Study the drawing (mm; zero at the part's minimum x, y, z) and answer. Round coordinates to 2 decimals unless told otherwise and drop trailing zeros. Loops run counter-clockwise (first coordinate to the right, second up) from the corner with the lowest first, then second, coordinate; pieces in that order, holes last. Notation, with made-up numbers: M -34.75,42 L -11.75,42 A6 ccw -11.75,49 Z; hole C 6.5,73 d5. An arc over 180 degrees is marked long. Put each result on its own line as item: value. Start each with the question number.
(1) Straight lines are drawn through the part: line 1 (X direction, y = 3.55, z = 130); line 2 (X direction, y = 3.2, z = 143.5); line 3 (Z direction, x = 28.5, y = 0.4). For each, find the intervals that lie inside material, in ascending order.
(2) Section C-C, the plane x = 22.5 is taken. Determine the outline of the cut face in (y, z).
(3) Section D-D, the plane x = 28.25 is taken. Determine the outline of the cut face in (y, z).
(4) Section A-A, the plane z = 130 is taken. Determine the outline of the cut face in (x, y), then the cut area to 3 significant figures.
(5) A flat-ended cylindrical pin translates along its axis: P1, Ø4.5, axis at x = 22.5, z = 115, coming from the +Y side. Find the tip coordinate at first contact, or state that the pin passes through.
(6) Section B-B, the plane y = 2.8 is taken. Count the separate pieces of the cut face and the enclosed holes in it, then the cut area to 3 significant figures.
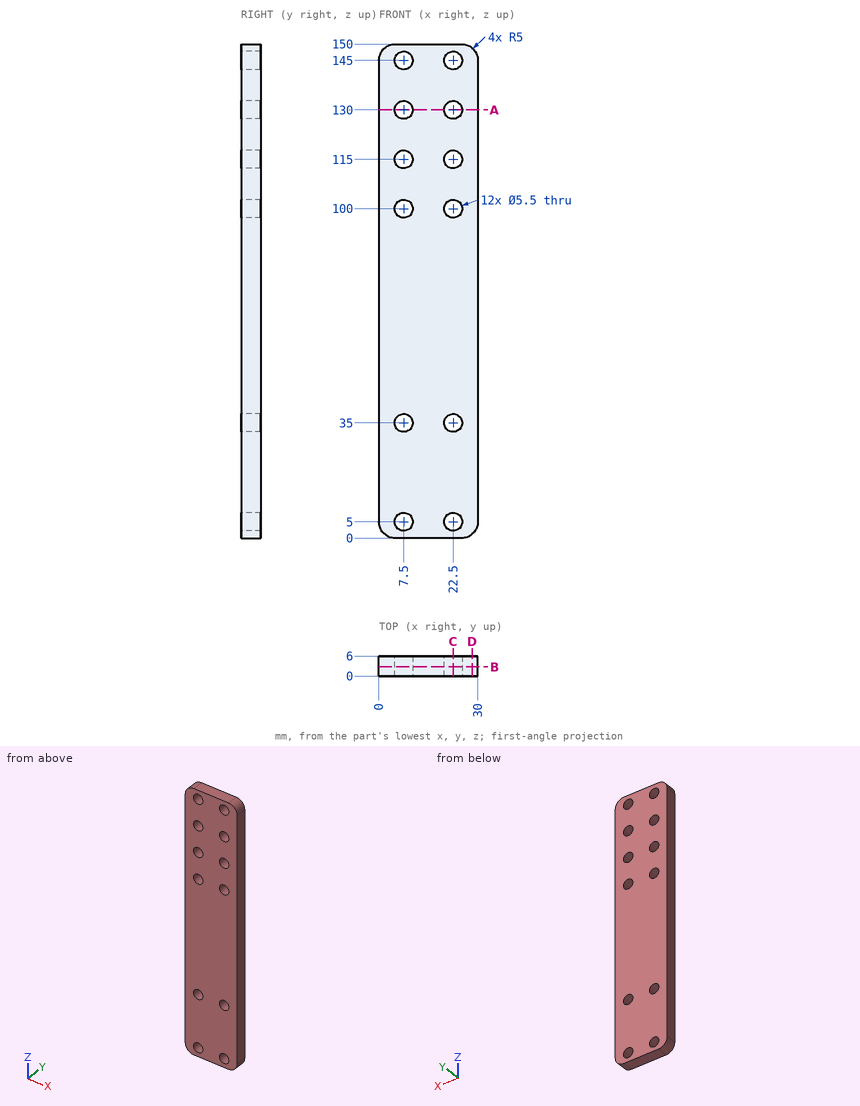
Recorded:
1. line 1: x = 0 to 4.75, 10.25 to 19.75, 25.25 to 30
1. line 2: x = 0 to 5.2, 9.8 to 20.2, 24.8 to 30
1. line 3: z = 1.43 to 148.57
2. outline: M 0,0 L 6,0 L 6,2.25 L 0,2.25 Z; M 0,7.75 L 6,7.75 L 6,32.25 L 0,32.25 Z; M 0,37.75 L 6,37.75 L 6,97.25 L 0,97.25 Z; M 0,102.75 L 6,102.75 L 6,112.25 L 0,112.25 Z; M 0,117.75 L 6,117.75 L 6,127.25 L 0,127.25 Z; M 0,132.75 L 6,132.75 L 6,142.25 L 0,142.25 Z; M 0,147.75 L 6,147.75 L 6,150 L 0,150 Z
3. outline: M 0,1.2 L 6,1.2 L 6,148.8 L 0,148.8 Z
4. outline: M 0,0 L 4.75,0 L 4.75,6 L 0,6 Z; M 10.25,0 L 19.75,0 L 19.75,6 L 10.25,6 Z; M 25.25,0 L 30,0 L 30,6 L 25.25,6 Z
4. area: 114 mm²
5. P1: passes through
6. separate pieces: 1
6. enclosed holes: 12
6. area: 4,190 mm²
